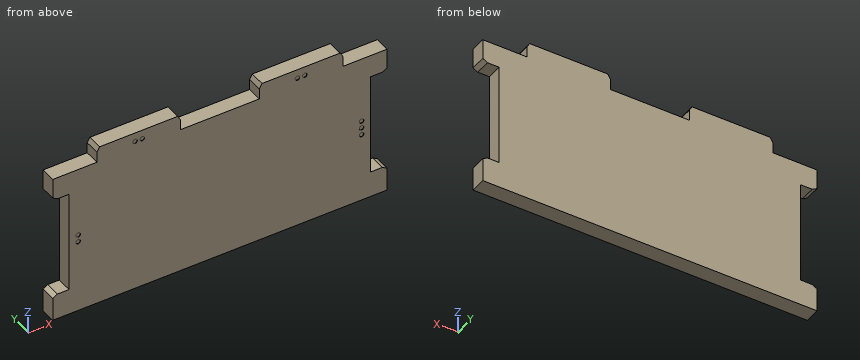
```python
from build123d import *

# Parameters (mm, degrees)
SKETCH1_W             = 93.653112922
SKETCH1_H             = 50
BOSS_EXTRUDE1_DEPTH   = 4.318
SKETCH3_W             = 23.386037641
SKETCH3_H             = 4.318
BOSS_EXTRUDE2_DEPTH   = 4.318
CUT_EXTRUDE1_REACH    = 6.318
SKETCH4_W             = 4.572
SKETCH4_H             = 28.575
CUT_EXTRUDE2_REACH    = 6.318
SKETCH5_W             = 93.653112922
SKETCH5_H             = 7.747
SKETCH8_R             = 0.635
CUT_EXTRUDE4_DEPTH    = 0.127
CHAMFER1_SIZE         = 0.762
CHAMFER1_SIZE2        = 1.319822715
CHAMFER1_PART_2_SIZE  = 0.762
CHAMFER1_PART_2_SIZE2 = 1.319822715
CHAMFER1_PART_3_SIZE  = 0.762
CHAMFER1_PART_3_SIZE2 = 1.319822715
CHAMFER1_PART_4_SIZE  = 0.762
CHAMFER1_PART_4_SIZE2 = 1.319822715
CHAMFER2_SIZE         = 0.762
CHAMFER2_SIZE2        = 1.319822715
CHAMFER2_PART_2_SIZE  = 0.762
CHAMFER2_PART_2_SIZE2 = 1.319822715
CHAMFER2_PART_3_SIZE  = 0.762
CHAMFER2_PART_3_SIZE2 = 1.319822715
CHAMFER2_PART_4_SIZE  = 0.762
CHAMFER2_PART_4_SIZE2 = 1.319822715


with BuildPart() as part:
    # Sketch1 → Boss-Extrude1 (new body)
    with BuildSketch(Plane(origin=(0, 0, 0), x_dir=(1, 0, 0), z_dir=(0, 1, 0))):
        Rectangle(SKETCH1_W, SKETCH1_H)
    extrude(amount=BOSS_EXTRUDE1_DEPTH)

    # Sketch3 → Boss-Extrude2 (add)
    with BuildSketch(Plane.XZ):
        with Locations((-22.751037641, 27.159)):
            Rectangle(SKETCH3_W, SKETCH3_H)
        with Locations((22.751037641, 27.159)):
            Rectangle(SKETCH3_W, SKETCH3_H)
    extrude(amount=-BOSS_EXTRUDE2_DEPTH)

    # Sketch4 → Cut-Extrude1 (cut, up to next)
    with BuildSketch(Plane(origin=(0, 4.318, 0), x_dir=(1, 0, 0), z_dir=(0, 1, 0)), mode=Mode.PRIVATE) as cut_extrude1_sk1:
        with Locations((-44.540556461, -4.3625)):
            Rectangle(SKETCH4_W, SKETCH4_H)
    cut_extrude1_tool1 = extrude(cut_extrude1_sk1.sketch, amount=-CUT_EXTRUDE1_REACH, mode=Mode.PRIVATE) & part.part
    add(cut_extrude1_tool1.solids().sort_by_distance((-44.540556, 4.318, 4.3625))[0], mode=Mode.SUBTRACT)
    # Sketch4 → Cut-Extrude1 (cut, up to next)
    with BuildSketch(Plane(origin=(0, 4.318, 0), x_dir=(1, 0, 0), z_dir=(0, 1, 0)), mode=Mode.PRIVATE) as cut_extrude1_sk2:
        with Locations((44.540556461, -4.3625)):
            Rectangle(SKETCH4_W, SKETCH4_H)
    cut_extrude1_tool2 = extrude(cut_extrude1_sk2.sketch, amount=-CUT_EXTRUDE1_REACH, mode=Mode.PRIVATE) & part.part
    add(cut_extrude1_tool2.solids().sort_by_distance((44.540556, 4.318, 4.3625))[0], mode=Mode.SUBTRACT)

    # Sketch5 → Cut-Extrude2 (cut, up to next)
    with BuildSketch(Plane(origin=(0, 4.318, 0), x_dir=(1, 0, 0), z_dir=(0, 1, 0)), mode=Mode.PRIVATE) as cut_extrude2_sk1:
        with Locations((0, 21.1265)):
            Rectangle(SKETCH5_W, SKETCH5_H)
    cut_extrude2_tool1 = extrude(cut_extrude2_sk1.sketch, amount=-CUT_EXTRUDE2_REACH, mode=Mode.PRIVATE) & part.part
    add(cut_extrude2_tool1.solids().sort_by_distance((0, 4.318, -21.1265))[0], mode=Mode.SUBTRACT)

    # Sketch8 → Cut-Extrude4 (cut)
    with BuildSketch(Plane.XZ):
        with Locations((21.735037641, 26.778)):
            Circle(SKETCH8_R)
        with Locations((23.767037641, 26.778)):
            Circle(SKETCH8_R)
        with Locations((39.714556461, 6.3945)):
            Circle(SKETCH8_R)
        with Locations((39.714556461, 4.3625)):
            Circle(SKETCH8_R)
        with Locations((39.714556461, 2.3305)):
            Circle(SKETCH8_R)
        with Locations((-23.767037641, 26.778)):
            Circle(SKETCH8_R)
        with Locations((-21.735037641, 26.778)):
            Circle(SKETCH8_R)
        with Locations((-39.714556461, 5.3785)):
            Circle(SKETCH8_R)
        with Locations((-39.714556461, 3.3465)):
            Circle(SKETCH8_R)
    extrude(amount=-CUT_EXTRUDE4_DEPTH, mode=Mode.SUBTRACT)

    # Chamfer1
    chamfer1_edges = [part.edges().sort_by_distance(p)[0] for p in [
        (-34.444056461, 2.159, 29.318),
    ]]
    chamfer1_side = [part.faces().sort_by_distance(p)[0] for p in [
        (-22.751037641, 2.159, 29.318),
    ]]
    chamfer(chamfer1_edges, length=CHAMFER1_SIZE, length2=CHAMFER1_SIZE2, reference=chamfer1_side[0])

    # Chamfer1 part 2
    chamfer1_part_2_edges = [part.edges().sort_by_distance(p)[0] for p in [
        (11.05801882, 2.159, 29.318),
    ]]
    chamfer1_part_2_side = [part.faces().sort_by_distance(p)[0] for p in [
        (22.751037641, 2.159, 29.318),
    ]]
    chamfer(chamfer1_part_2_edges, length=CHAMFER1_PART_2_SIZE, length2=CHAMFER1_PART_2_SIZE2, reference=chamfer1_part_2_side[0])

    # Chamfer1 part 3
    chamfer1_part_3_edges = [part.edges().sort_by_distance(p)[0] for p in [
        (-46.826556461, 2.159, -9.925),
    ]]
    chamfer1_part_3_side = [part.faces().sort_by_distance(p)[0] for p in [
        (-46.826556461, 2.159, -13.589),
    ]]
    chamfer(chamfer1_part_3_edges, length=CHAMFER1_PART_3_SIZE, length2=CHAMFER1_PART_3_SIZE2, reference=chamfer1_part_3_side[0])

    # Chamfer1 part 4
    chamfer1_part_4_edges = [part.edges().sort_by_distance(p)[0] for p in [
        (46.826556461, 2.159, 18.65),
    ]]
    chamfer1_part_4_side = [part.faces().sort_by_distance(p)[0] for p in [
        (46.826556461, 2.159, 21.825),
    ]]
    chamfer(chamfer1_part_4_edges, length=CHAMFER1_PART_4_SIZE, length2=CHAMFER1_PART_4_SIZE2, reference=chamfer1_part_4_side[0])

    # Chamfer2
    chamfer2_edges = [part.edges().sort_by_distance(p)[0] for p in [
        (-11.05801882, 2.159, 29.318),
    ]]
    chamfer2_side = [part.faces().sort_by_distance(p)[0] for p in [
        (-22.370037641, 2.159, 29.318),
    ]]
    chamfer(chamfer2_edges, length=CHAMFER2_SIZE, length2=CHAMFER2_SIZE2, reference=chamfer2_side[0])

    # Chamfer2 part 2
    chamfer2_part_2_edges = [part.edges().sort_by_distance(p)[0] for p in [
        (34.444056461, 2.159, 29.318),
    ]]
    chamfer2_part_2_side = [part.faces().sort_by_distance(p)[0] for p in [
        (23.132037641, 2.159, 29.318),
    ]]
    chamfer(chamfer2_part_2_edges, length=CHAMFER2_PART_2_SIZE, length2=CHAMFER2_PART_2_SIZE2, reference=chamfer2_part_2_side[0])

    # Chamfer2 part 3
    chamfer2_part_3_edges = [part.edges().sort_by_distance(p)[0] for p in [
        (-46.826556461, 2.159, 18.65),
    ]]
    chamfer2_part_3_side = [part.faces().sort_by_distance(p)[0] for p in [
        (-46.826556461, 2.159, 21.825),
    ]]
    chamfer(chamfer2_part_3_edges, length=CHAMFER2_PART_3_SIZE, length2=CHAMFER2_PART_3_SIZE2, reference=chamfer2_part_3_side[0])

    # Chamfer2 part 4
    chamfer2_part_4_edges = [part.edges().sort_by_distance(p)[0] for p in [
        (46.826556461, 2.159, -9.925),
    ]]
    chamfer2_part_4_side = [part.faces().sort_by_distance(p)[0] for p in [
        (46.826556461, 2.159, -13.589),
    ]]
    chamfer(chamfer2_part_4_edges, length=CHAMFER2_PART_4_SIZE, length2=CHAMFER2_PART_4_SIZE2, reference=chamfer2_part_4_side[0])


solid = part.part
```
CAD build for the part. Positions are in the model's coordinates, mm. Round coordinates to 2 decimals unless told otherwise and drop trailing zeros. Write each loop counter-clockwise with the first axis right and the second up, starting at its lowest first coordinate (ties: lowest second). Pieces come first, ordered by that corner, then holes. Notation, with made-up numbers: (61, -39) - (97, -39) arc R22 cw to (97, -19) - close; hole circle Ø1 at (-7, 1). An arc over 180 degrees is marked (long way). Write item = value, one per line. Start each with the question number.
Q1. Band-saw the part on B-B (z = 17). Give the cut face in (x, y), then the cut area to 3 significant figures.
Q2. Drop flat-ended pins along their axis: pin 1 (3 mm diameter, centred on x = 30, z = -4.5, fed in from -Y); pin 2 (2 mm diameter, centred on y = 1, z = 10.5, fed in from +X); pin 3 (0.8 mm diameter, centred on x = -39.71, z = 3.35, fed in from -Y); pin 4 (2 mm diameter, centred on x = 39, y = 1.5, fed in from +Z). Give the stop position or say it passes through.
Q3. Band-saw the part on C-C (x = 7). Give the cut face in (y, z).
Q4. Band-saw the part on A-A (y = 1.4). Give the cut face in (x, z) (3 decimals).
Q5. Probe L1, parallel to X at y = 1.95, z = 25.5; L2, parallel to X at y = 0.45, z = 8; L3, parallel to Z at x = -43, y = 2.9 (3 decimals). List the from-to ranges inside material, lowest first. Write a range as from..to.
Answers below:
q1.outline = (-42.25, 0) - (42.25, 0) - (42.25, 4.32) - (-42.25, 4.32) - close
q1.area = 365 mm2
q2.pin_1 = 0
q2.pin_2 = 42.25
q2.pin_3 = 0.13
q2.pin_4 = 25
q3.outline = (0, -17.25) - (4.32, -17.25) - (4.32, 25) - (0, 25) - close
q4.outline = (-46.827, -17.253) - (46.827, -17.253) - (46.827, -10.687) - (45.507, -9.925) - (42.255, -9.925) - (42.255, 18.65) - (45.507, 18.65) - (46.827, 19.412) - (46.827, 25) - (34.444, 25) - (34.444, 27.998) - (33.682, 29.318) - (11.82, 29.318) - (11.058, 27.998) - (11.058, 25) - (-11.058, 25) - (-11.058, 27.998) - (-11.82, 29.318) - (-33.682, 29.318) - (-34.444, 27.998) - (-34.444, 25) - (-46.827, 25) - (-46.827, 19.412) - (-45.507, 18.65) - (-42.255, 18.65) - (-42.255, -9.925) - (-45.507, -9.925) - (-46.827, -10.687) - close
q5.L1 = -34.44..-11.06, 11.06..34.44
q5.L2 = -42.25..42.25
q5.L3 = -17.253..-9.925, 18.65..25
